```python
from build123d import *

# Parameters (mm, degrees)
SKETCH1_R           = 23.6982
SKETCH1_R_2         = 22.225
BOSS_EXTRUDE1_DEPTH = 635
CUT_EXTRUDE1_START  = -77.831769
SKETCH2_W           = 3.175
SKETCH2_H           = 98.425
CUT_EXTRUDE1_DEPTH  = 1.529969
CIRPATTERN2_COUNT   = 3


with BuildPart() as part:
    # Sketch1 → Boss-Extrude1 (new body)
    with BuildSketch(Plane.XY):
        Circle(SKETCH1_R)
        Circle(SKETCH1_R_2, mode=Mode.SUBTRACT)
    extrude(amount=BOSS_EXTRUDE1_DEPTH)

    # Sketch2 → Cut-Extrude1 (cut)
    with BuildSketch(Plane(origin=(0, 100, 0), x_dir=(1, 0, 0), z_dir=(0, 1, 0)).offset(CUT_EXTRUDE1_START)):
        with Locations((0, -493.7125)):
            Rectangle(SKETCH2_W, SKETCH2_H)
    cut_extrude1 = extrude(amount=CUT_EXTRUDE1_DEPTH, mode=Mode.SUBTRACT)

    # CirPattern2: Cut-Extrude1 ×3 about axis
    cirpattern2_axis = Axis((0, 0, 0), (0, 0, 1))
    for i in range(1, CIRPATTERN2_COUNT):
        add(cut_extrude1.rotate(cirpattern2_axis, i * 360 / CIRPATTERN2_COUNT), mode=Mode.SUBTRACT)


solid = part.part
```
Part model, mm, in its own coordinate system. Coordinates: 2 decimals unless noted, no trailing zeros. Order: outer loops, then holes, each group sorted by start corner. A loop starts at its lowest first (then second) coordinate and runs counter-clockwise, first axis right, second up. Notation, with made-up numbers: (-15.75, 67.5) - (41.25, 67.5) arc R18 ccw to (41.25, 75.5) - close; hole circle Ø6 at (57.25, 74.5). An arc over 180 degrees is marked (long way). Return JSON: item names as keys, results as strings. Group by question number.
Item 1: Cut at C-C (z = 269). List the corners of the cut face in (x, y) (3 decimals), plus the area to 3 significant figures.
Item 2: Pull direction Y, two halves, no side cores. Call faces 1 (the face through (21.199, 6.676, 313.055)), 2 (the face through (-5.137, -23.135, 313.055)): pulls with the +Y half, pulls with the -Y half, needs draft (parallel to the pull), parting line crosses it, or undercut.
Item 3: Drill centre lines: probe 1 along X at (y, z) = (2, 164.5); probe 2 along Y at (x, z) = (0, 419.5) (3 decimals); probe 3 along Y at (x, z) = (-9, 121.5). Where is each one in solid material? Low to high. Write a range as from..to.
Item 4: Pin check, flat tips, straight feed: pin 1 (10 mm diameter, centred on y = -15, z = 205, fed in from +X) (3 decimals); pin 2 (1.4 mm diameter, centred on x = 19, y = -11, fed in from +Z); pin 3 (4 mm diameter, centred on y = -15.5, z = 146, fed in from +X); pin 4 (6 mm diameter, centred on x = 14, z = 422.5, fed in from -Y). Stop position of each tip, or through.
Item 5: Cut at A-A (y = 0). List the corners of the cut face in (x, z) (3 decimals), plus the area to 3 significant figures.
Item 6: Cut at B-B (x = -7). List the corners of the cut face in (y, z).
Check values:
{
 "1": {"outline": "circle Ø47.396 at (0, 0); hole circle Ø44.45 at (0, 0)", "area": "213 mm2"},
 "2": {"face 1": "undercut", "face 2": "parting line crosses it"},
 "3": {"probe 1": "x = -23.61..-22.13, 22.13..23.61", "probe 2": "y = -23.698..-22.225, 22.225..23.698", "probe 3": "y = -21.92..-20.32, 20.32..21.92"},
 "4": {"pin 1": "stops at x = 21.485", "pin 2": "stops at z = 635", "pin 3": "stops at x = 19.48", "pin 4": "stops at y = -20.99"},
 "5": {"outline": "(-23.698, 0) - (-22.225, 0) - (-22.225, 635) - (-23.698, 635) - close; (22.225, 0) - (23.698, 0) - (23.698, 635) - (22.225, 635) - close", "area": "1,870 mm2"},
 "6": {"outline": "(-22.64, 0) - (-21.09, 0) - (-21.09, 635) - (-22.64, 635) - close; (21.09, 0) - (22.64, 0) - (22.64, 635) - (21.09, 635) - close"}
}
